Verification items for the finished model (mm, model axes). Face numbers are marked on the shaded views. Coordinates: 2 decimals unless noted, no trailing zeros. Write each loop counter-clockwise with the first axis right and the second up, starting at its lowest first coordinate (ties: lowest second). Pieces come first, ordered by that corner, then holes. Notation, with made-up numbers: (7, -37.75) -> (21, -37.75) arc R12 ccw to (21, -16.75) -> close; hole circle Ø9 at (36.5, 24). An arc over 180 degrees is marked (long way). Write item = value, one per line. Start each with the question number.
(1) Section check D-D (y = 13). Record the cut outline in (x, z).
(2) Gauge pin test, flat ends, axial feed: pin 1 Ø4 at (x, y) = (8, 7) entering from -Z; pin 2 Ø3 at (x, y) = (3, -14.5) entering from +Z; pin 3 Ø12 at (y, z) = (-13.5, -0.5) entering from -X. Record the tip position at first contact, or that the pin passes through.
(3) Section check A-A (y = 7). Record the cut outline in (x, z), plus the area to 3 significant figures.
(4) Section check C-C (x = -16). Record the cut outline in (y, z).
(5) Material ranges on probe 1 along Y at (x, z) = (-5.5, -9); probe 2 along Y at (x, z) = (14, 15); probe 3 along X at (y, z) = (-10.5, -13), recorded low to high. Write a range as [from, to].
(6) Section check B-B (z = -12). Record the cut outline in (x, y), plus the area to 3 significant figures.
(7) Mould release check, pull along Z, two halves, no side actions. Record for the marked faces 1 and 2: released by +Z, released by -Z, zero draft, split by the parting line, or undercut.
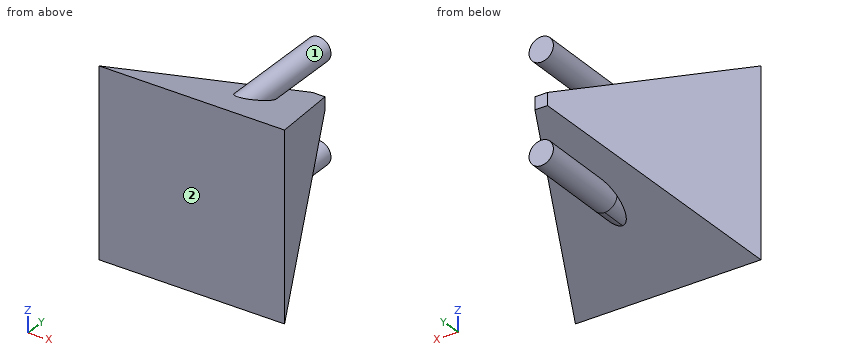
```python
from build123d import *

# Parameters (mm, degrees)
SKETCH1_W           = 38.1
SKETCH1_H           = 38.1
BOSS_EXTRUDE1_DEPTH = 19.05
DRAFT1_ANGLE        = -25
SKETCH2_R           = 2.5
BOSS_EXTRUDE3_DEPTH = 19.05


with BuildPart() as part:
    # Sketch1 → Boss-Extrude1 (new, symmetric)
    with BuildSketch(Plane(origin=(0, 0, 0), x_dir=(1, 0, 0), z_dir=(0, 1, 0))):
        Rectangle(SKETCH1_W, SKETCH1_H)
    extrude(amount=BOSS_EXTRUDE1_DEPTH, both=True)

    # Draft1
    draft1_faces = [part.faces().sort_by_distance(p)[0] for p in [
        (-19.05, 0, 0),
        (0, 0, 19.05),
        (19.05, 0, 0),
        (0, 0, -19.05),
    ]]
    draft(draft1_faces, Plane(origin=(0, -19.05, 0), x_dir=(0, 0, -1), z_dir=(0, -1, 0)), DRAFT1_ANGLE)

    # Sketch2 → Boss-Extrude3 (add, symmetric)
    with BuildSketch(Plane(origin=(0, 0, 0), x_dir=(1, 0, 0), z_dir=(0, 1, 0))):
        with Locations(Location((0, 10.166839112, 0), (0, 0, 90))):
            Circle(SKETCH2_R)
        with Locations(Location((0, -10.166839112, 0), (0, 0, 90))):
            Circle(SKETCH2_R)
    extrude(amount=BOSS_EXTRUDE3_DEPTH, both=True)


solid = part.part
```
Response:
q1.outline = (-4.1, -4.1) -> (4.1, -4.1) -> (4.1, 4.1) -> (-4.1, 4.1) -> close; circle Ø5 at (0, -10.17); circle Ø5 at (0, 10.17)
q2.pin_1 = -7.83
q2.pin_2 = 17.63
q2.pin_3 = -19.05
q3.outline = (-6.9, -6.9) -> (6.9, -6.9) -> (6.9, 6.9) -> (-6.9, 6.9) -> close; circle Ø5 at (0, -10.17); circle Ø5 at (0, 10.17)
q3.area = 230 mm2
q4.outline = (-19.05, -19.05) -> (-12.51, -16) -> (-12.51, 16) -> (-19.05, 19.05) -> close
q5.probe_1 = [-19.05, 2.5]
q5.probe_2 = [-19.05, -10.36]
q5.probe_3 = [-15.06, 15.06]
q6.outline = (-19.05, -19.05) -> (19.05, -19.05) -> (12, -3.93) -> (1.7, -3.93) -> (1.7, 19.05) -> (-1.7, 19.05) -> (-1.7, -3.93) -> (-12, -3.93) -> close
q6.area = 548 mm2
q7.face_1 = undercut
q7.face_2 = zero draft
